Here's the drawing with two shaded views (mm, measured from the low corner). I have some questions. A direction names the side the tool comes from. Give positions to 0.01 mm unless a question says otherwise; leave off trailing zeros. Write each loop counter-clockwise with the first axis right and the second up, starting at its lowest first coordinate (ties: lowest second). Pieces come first, ordered by that corner, then holes. Notation, with made-up numbers: (8, 16.25) -> (64, 16.25) arc R5 cw to (64, 24.25) -> close; hole circle Ø11 at (-32.5, -4.5). An arc over 180 degrees is marked (long way). One line per question, with ' | ' between items.
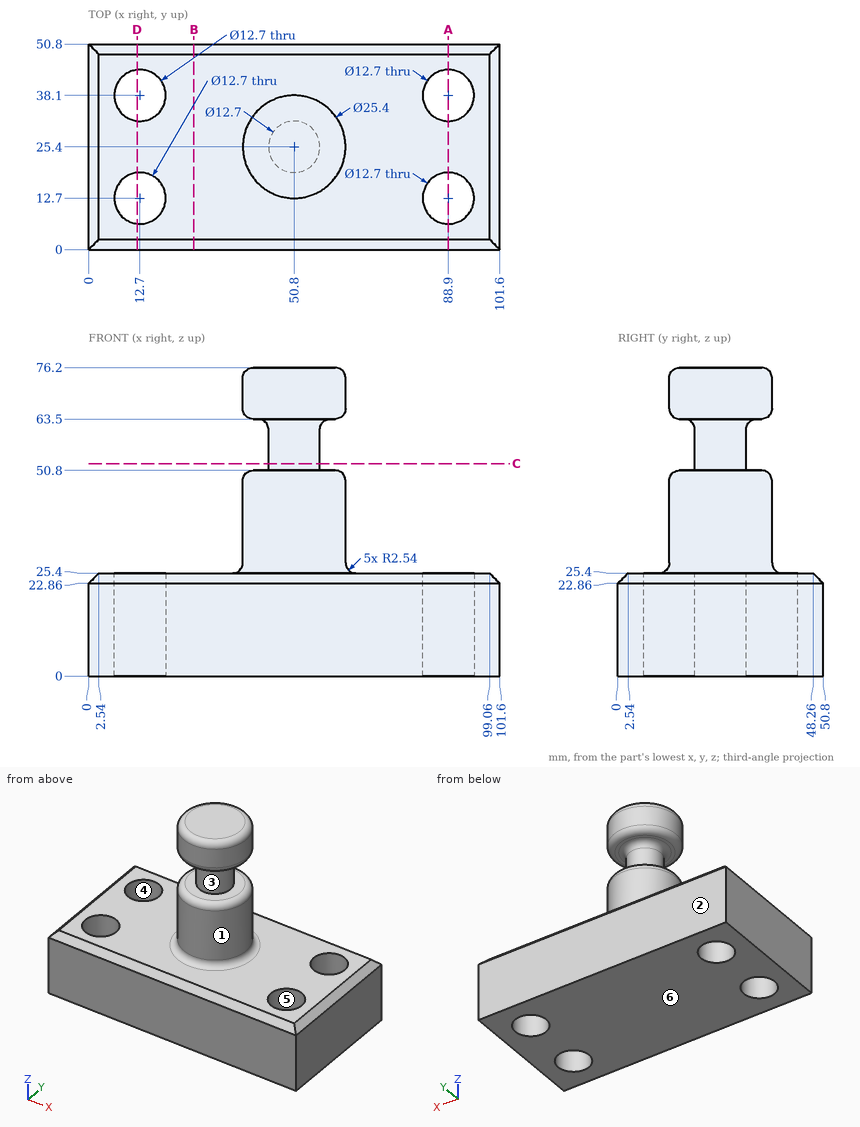
Q1. Imagine slicing it at B-B on x = 26. Please give me the cut outline in (y, z), and give its area (3 significant figures).
Answer below:
outline: (0, 0) -> (50.8, 0) -> (50.8, 22.86) -> (48.26, 25.4) -> (2.54, 25.4) -> (0, 22.86) -> close | area: 1,280 mm^2
Q2. Imagine slicing it at D-D on x = 12. Please give me the cut outline in (y, z), and give its area (3 significant figures).
Answer below:
outline: (0, 0) -> (6.39, 0) -> (6.39, 25.4) -> (2.54, 25.4) -> (0, 22.86) -> close; (19.01, 0) -> (31.79, 0) -> (31.79, 25.4) -> (19.01, 25.4) -> close; (44.41, 0) -> (50.8, 0) -> (50.8, 22.86) -> (48.26, 25.4) -> (44.41, 25.4) -> close | area: 643 mm^2
Q3. Imagine slicing it at A-A on x = 88.9. Please give me the cut outline in (y, z), and give its area (3 significant figures).
Answer below:
outline: (0, 0) -> (6.35, 0) -> (6.35, 25.4) -> (2.54, 25.4) -> (0, 22.86) -> close; (19.05, 0) -> (31.75, 0) -> (31.75, 25.4) -> (19.05, 25.4) -> close; (44.45, 0) -> (50.8, 0) -> (50.8, 22.86) -> (48.26, 25.4) -> (44.45, 25.4) -> close | area: 639 mm^2
Q4. If I drill on line 1 along X through (y, z) = (12.5, 7.5); line 2 along Y through (x, z) = (12.7, 16.5); line 3 along X through (y, z) = (35.5, 11), over which ranges is the centre line in solid material (lowest first)?
Answer below:
line 1: x = 0 to 6.35, 19.05 to 82.55, 95.25 to 101.6 | line 2: y = 0 to 6.35, 19.05 to 31.75, 44.45 to 50.8 | line 3: x = 0 to 6.91, 18.49 to 83.11, 94.69 to 101.6
Q5. Will these pins go through, and if not, where does the flat tip stop? pin 1 (11.5 mm diameter, centred on x = 88.9, y = 38.1, fed in from +Z); pin 2 (1.5 mm diameter, centred on x = 83.5, y = 18, fed in from +Z); pin 3 (3 mm diameter, centred on y = 29, z = 53, fed in from -X).
Answer below:
pin 1: passes through | pin 2: stops at z = 25.4 | pin 3: stops at x = 44.81
Q6. If we mould it in two halves opening along Y, with no side actions, what happens to the marked faces 3, 4, 5 and 6? For each: +Y half, -Y half, draft (parallel to the pull), parting line (faces both ways), or undercut.
Answer below:
face 3: parting line | face 4: undercut | face 5: undercut | face 6: draft
Q7. Imagine slicing it at C-C on z = 52.5. Please give me the cut outline in (x, y).
Answer below:
outline: circle Ø12.7 at (50.8, 25.4)
Q8. On a 3-axis mill with a long thin cutter (end or side, diameter ignored), from which of +Z, -Z, +X, -X, +Y, -Y can I reach the whole of each face in a straight line? I mean the marked faces 1 and 2. Say none if no direction works.
Answer below:
face 1: +Z | face 2: +Z, -Z, +X, -X, +Y
